from build123d import *

# Parameters (mm, degrees)
SKETCH1_W           = 25.4
SKETCH1_H           = 25.4
BOSS_EXTRUDE2_DEPTH = 609.6
SKETCH2_W           = 20.302766191
SKETCH2_H           = 19.05
CUT_EXTRUDE1_DEPTH  = 611.657416233
CUT_EXTRUDE2_DEPTH  = 611.657416233


with BuildPart() as part:
    # Sketch1 → Boss-Extrude2 (new body)
    with BuildSketch(Plane.XY):
        with Locations((12.7, 12.7)):
            Rectangle(SKETCH1_W, SKETCH1_H)
    extrude(amount=BOSS_EXTRUDE2_DEPTH)

    # Sketch2 → Cut-Extrude1 (cut, through all)
    with BuildSketch(Plane(origin=(0, 0, 0), x_dir=(-1, 0, 0), z_dir=(0, 0, -1))):
        with Locations((-13.326383096, 12.7)):
            Rectangle(SKETCH2_W, SKETCH2_H)
    extrude(amount=-CUT_EXTRUDE1_DEPTH, mode=Mode.SUBTRACT)

    # Sketch3 → Cut-Extrude2 (cut, through all)
    with BuildSketch(Plane(origin=(25.4, 0, 0), x_dir=(0, 0, -1), z_dir=(1, 0, 0))):
        Polygon((0, 25.4), (-25.4, 0), (0, 0), align=None)
    extrude(amount=-CUT_EXTRUDE2_DEPTH, mode=Mode.SUBTRACT)


solid = part.part
Design review of the part built by this model. Coordinates are the model's own, in mm. A direction names the side the tool comes from. Round coordinates to 2 decimals unless told otherwise and drop trailing zeros. Write each loop counter-clockwise with the first axis right and the second up, starting at its lowest first coordinate (ties: lowest second). Pieces come first, ordered by that corner, then holes.
Item 1: Draft analysis for pull direction X (two halves, no side actions). For faces 3 (the flat face through (3.175, 13, 302)), 4 (the flat face through (25.4, 13, 301)), 5 (the flat face through (0, 13, 301)), 6 (the flat face through (1.6, 12.9, 12.5)), state which applies: released by +X, released by -X, zero draft, split by the parting line, or undercut.
Item 2: Consider section B-B on x = 15.75. Give the boundary of the cut face in (y, z) (3 decimals).
Item 3: Consider section A-A on y = 12.25. Give the boundary of the cut face in (x, z) (3 decimals), and give its area (3 significant figures).
Item 4: For pin 1 Ø6 at (x, z) = (12, 446.5) entering from -Y; pin 2 Ø3 at (x, y) = (21.5, 12) entering from +Z, all flat-tipped, find the tip position at first contact; note any pin that passes through.
Item 5: For faces 1 (the flat face through (13, 0, 313)), 2 (the flat face through (13, 22.225, 302)), list the 3-axis set-ups (+Z, -Z, +X, -X, +Y, -Y) from which the entire face can be reached by the end or side of a thin tool; tool diameter is ignored.
Item 6: Wall thickness on L1, parallel to Y at x = 11.5, z = 97.5 (3 decimals); L2, parallel to X at y = 17.5, z = 463 (3 decimals); L3, parallel to Z at x = 1, y = 2: over which ranges is each line inside the solid? List them lowest first.
Item 7: Consider section C-C on z = 283. Give the boundary of the cut face in (x, y) (3 decimals).
Check values:
1. face 3: undercut
1. face 4: released by +X
1. face 5: released by -X
1. face 6: zero draft
2. outline: (0, 25.4) - (3.175, 22.225) - (3.175, 609.6) - (0, 609.6) - close; (22.225, 3.175) - (25.4, 0) - (25.4, 609.6) - (22.225, 609.6) - close
3. outline: (0, 13.15) - (3.175, 13.15) - (3.175, 609.6) - (0, 609.6) - close; (23.478, 13.15) - (25.4, 13.15) - (25.4, 609.6) - (23.478, 609.6) - close
3. area: 3,040 mm2
4. pin 1: stops at y = 0
4. pin 2: passes through
5. face 1: +Z, -Z, +X, -X, -Y
5. face 2: +Z, -Z
6. L1: y = 0 to 3.175, 22.225 to 25.4
6. L2: x = 0 to 3.175, 23.478 to 25.4
6. L3: z = 23.4 to 609.6
7. outline: (0, 0) - (25.4, 0) - (25.4, 25.4) - (0, 25.4) - close; hole (3.175, 3.175) - (23.478, 3.175) - (23.478, 22.225) - (3.175, 22.225) - close
